Input: part model. Units: mm. Frame: model coordinates. Face numbers are marked on the shaded views. Round coordinates to 2 decimals unless told otherwise and drop trailing zeros. Loops run counter-clockwise (first coordinate to the right, second up) from the corner with the lowest first, then second, coordinate; pieces in that order, holes last.
(1) Cut plane A-A, the plane x = -8. Output: boundary loops of the cut face in (y, z).
(2) Line query: line 1 (X direction, y = 4, z = 5); line 2 (X direction, y = -4.75, z = -4); line 3 (Z direction, x = 23.1, y = 0). Output: solid intervals per line, ascending.
(3) First-contact query: pin 1 Ø8 at (y, z) = (0, 0) entering from +X; pin 2 Ø4.5 at (y, z) = (-0.5, 1) entering from -X; pin 3 Ø4.5 at (y, z) = (0, 0) entering from -X. Flat tips, straight axial feed; report the tip coordinate or a pass-through.
(4) Draft query along Z for the marked faces 1 and 2. Return one class per face: released by +Z, released by -Z, zero draft, split by the parting line, or undercut.
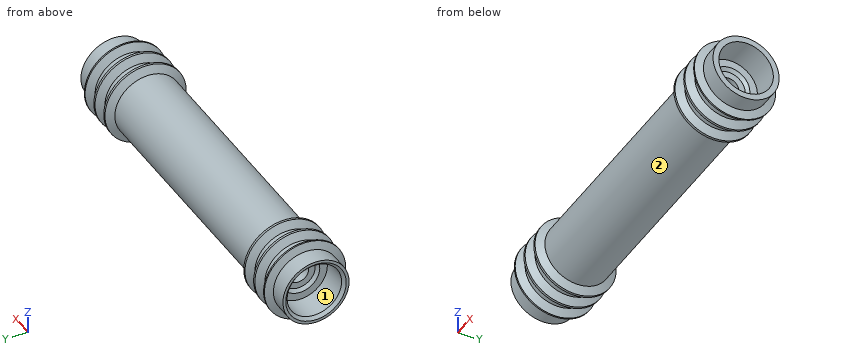
from build123d import *

# Parameters (mm, degrees)
CHAMFER1_SIZE = 0.508


with BuildPart() as part:
    # Sketch2 → Revolve1 (revolve)
    with BuildSketch(Plane.XY, mode=Mode.PRIVATE) as revolve1_sk:
        Polygon((-28.75, 5.55625), (-31.75, 5.55625), (-31.75, 4.575), (-26.75, 4.575), (-26.75, 3.305), (-26.242, 2.797), (-26.242, 1.7145), (-21.925, 1.7145), (-21.925, 0), (0, 0), (0, 3.175), (0, 5.55625), (-21.070060633, 5.55625), (-21.803295474, 6.82625), (-22.184295474, 6.82625), (-22.917530316, 5.55625), (-24.187530316, 5.55625), (-24.920765158, 6.82625), (-25.301765158, 6.82625), (-26.035, 5.55625), (-27.305, 5.55625), (-28.038234842, 6.82625), (-28.287757802, 6.82625), align=None)
    revolve(revolve1_sk.sketch.rotate(Axis((-31.75, 0, 0), (1, 0, 0)), 180), axis=Axis((-31.75, 0, 0), (1, 0, 0)))

    # Mirror1: part across plane


with BuildPart() as part_1:
    add(part.part)
    add(part.part.mirror(Plane(origin=(0, 0, 0), x_dir=(0, 0, 1), z_dir=(1, 0, 0))))

    # Chamfer1
    chamfer1_edges = [part_1.edges().sort_by_distance(p)[0] for p in [
        (-31.75, 4.575, 0),
    ]]
    chamfer(chamfer1_edges, length=CHAMFER1_SIZE)


solid = part_1.part
Reported:
1. outline: circle Ø11.11 at (0, 0)
2. line 1: x = -28.44 to -27.79, -25.55 to -24.68, -22.43 to -21.56, 21.56 to 22.43, 24.68 to 25.55, 27.79 to 28.44
2. line 2: x = -28.51 to -27.68, -25.66 to -24.56, -22.54 to -21.45, 21.45 to 22.54, 24.56 to 25.66, 27.68 to 28.51
2. line 3: z = -5.56 to -1.71, 1.71 to 5.56
3. pin 1: stops at x = 26.75
3. pin 2: stops at x = -26.75
3. pin 3: stops at x = -26.24
4. face 1: undercut
4. face 2: split by the parting line
